Input: part model. Units: mm. Frame: model coordinates. Face numbers are marked on the shaded views. A direction names the side the tool comes from. Round coordinates to 2 decimals unless told otherwise and drop trailing zeros. Loops run counter-clockwise (first coordinate to the right, second up) from the corner with the lowest first, then second, coordinate; pieces in that order, holes last. Notation, with made-up numbers: M -1,46 L 56,46 A24 cw 56,62 Z; hole C 88,22 d4. An arc over 180 degrees is marked long. Put each result on its own line as item: value. Start each with the question number.
1) Pin query (flat end, axial travel): pin 1 (1.9 mm diameter, centred on x = -6, z = -16, fed in from -Y); pin 2 (1.8 mm diameter, centred on y = 2.5, z = -1, fed in from +X); pin 3 (3.5 mm diameter, centred on x = 6, z = -16, fed in from +Y); pin 4 (6 mm diameter, centred on x = -9, z = 7, fed in from +Y). Return the tip coordinate at first contact, or that it passes through.
2) Draft query along Y for the marked faces 4, 5 and 6. Return one class per face: +Y half, -Y half, draft (parallel to the pull), parting line (faces both ways), or undercut.
3) Section B-B on x = 6. Output: boundary loops of the cut face in (y, z).
4) Reachability of the marked faces 1, 2 and 3 from +Z, -Z, +X, -X, +Y, -Y: full face, straight path, thin tool, end or side. Return the list, or none.
5) Section A-A on z = -16. Output: boundary loops of the cut face in (x, y).
6) Line query: probe 1 along X at (y, z) = (-0.55, -16); probe 2 along Z at (x, y) = (6, -0.25); probe 3 along Z at (x, y) = (6.5, 3). Output: solid intervals per line, ascending.
7) Section D-D on y = -0.5. Output: boundary loops of the cut face in (x, z), plus the area to 3 significant figures.
8) Section C-C on x = 3.5. Output: boundary loops of the cut face in (y, z), plus the area to 4 significant figures.
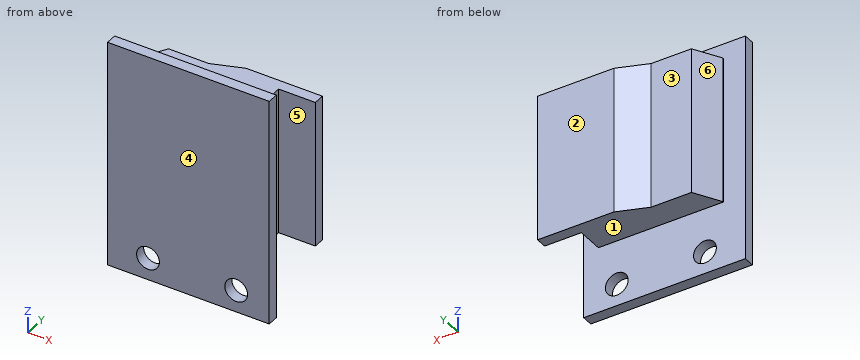
from build123d import *

# Parameters (mm, degrees)
SKIZZE2_W                        = 17
SKIZZE2_H                        = 20
AUFSATZ_LINEAR_AUSTRAGEN1_DEPTH  = 3.6
SKIZZE3_W                        = 22
SKIZZE3_H                        = 31
AUFSATZ_LINEAR_AUSTRAGEN2_DEPTH  = 1.5
F_3_1_3_1_DURCHMESSER_BOHRUNG1_D = 3.1
SKIZZE10_W                       = 10
SKIZZE10_H                       = 20
AUFSATZ_LINEAR_AUSTRAGEN3_DEPTH  = 1.5
FASE4_SIZE                       = 4.5
FASE4_SIZE_2                     = 1.637866054
FASE5_SIZE                       = 3.5
FASE5_SIZE2                      = 2.020725942


with BuildPart() as part:
    # Skizze2 → Aufsatz-Linear austragen1 (new body)
    with BuildSketch(Plane(origin=(0, 0, 0), x_dir=(1, 0, 0), z_dir=(0, 1, 0))):
        Rectangle(SKIZZE2_W, SKIZZE2_H)
    extrude(amount=AUFSATZ_LINEAR_AUSTRAGEN1_DEPTH)

    # Skizze3 → Aufsatz-Linear austragen2 (add)
    with BuildSketch(Plane(origin=(0, 0, 0), x_dir=(-1, 0, 0), z_dir=(0, -1, 0))):
        with Locations((0.5, 3.5)):
            Rectangle(SKIZZE3_W, SKIZZE3_H)
    extrude(amount=AUFSATZ_LINEAR_AUSTRAGEN2_DEPTH)

    # Ø3.1 (3.1) Durchmesser Bohrung1 (through all)
    with Locations(Plane(origin=(0, -1.5, 0), x_dir=(-1, 0, 0), z_dir=(0, -1, 0))):
        with Locations((6, 16), (-6, 16)):
            Hole(F_3_1_3_1_DURCHMESSER_BOHRUNG1_D / 2)

    # Skizze10 → Aufsatz-Linear austragen3 (add)
    with BuildSketch(Plane(origin=(0, 3.6, 0), x_dir=(1, 0, 0), z_dir=(0, 1, 0))):
        with Locations((8.5, 0)):
            Rectangle(SKIZZE10_W, SKIZZE10_H)
    extrude(amount=AUFSATZ_LINEAR_AUSTRAGEN3_DEPTH)

    # Fase4
    # the kernel refuses this chamfer: 4.5, 1.637866054 mm, written as the material it adds along each edge
    with BuildSketch(Plane(origin=(3.5, 3.6, -10), x_dir=(-0.9999130865277315, -0.01318405819864591, 0), z_dir=(0, 0, 1))) as fase4_piece_1_section:
        Polygon((FASE4_SIZE * 0.999913086528, -FASE4_SIZE * 0.0131840581986), (-FASE4_SIZE_2 * 0.0131840582002, -FASE4_SIZE_2 * 0.999913086649), (0, 0), align=None)
    fase4_piece_1 = extrude(amount=20, mode=Mode.PRIVATE)
    fase4_piece_1 = split(fase4_piece_1, bisect_by=Plane(origin=(1.935786974, 5.1, 0), z_dir=(0, -1, 0)), keep=Keep.TOP, mode=Mode.PRIVATE)
    add(fase4_piece_1)

    # Fase5
    fase5_edges = [part.edges().sort_by_distance(p)[0] for p in [
        (-8.5, 3.6, 0),
    ]]
    fase5_side = [part.faces().sort_by_distance(p)[0] for p in [
        (-8.5, 1.8, 0),
    ]]
    chamfer(fase5_edges, length=FASE5_SIZE, length2=FASE5_SIZE2, reference=fase5_side[0])


solid = part.part
Geometry results:
1. pin 1: passes through
1. pin 2: stops at x = 8.5
1. pin 3: stops at y = 0
1. pin 4: stops at y = 3.6
2. face 4: -Y half
2. face 5: undercut
2. face 6: +Y half
3. outline: M -1.5,-19 L 0,-19 L 0,-17.55 L -1.5,-17.55 Z; M -1.5,-14.45 L 0,-14.45 L 0,-10 L 5.1,-10 L 5.1,10 L 0,10 L 0,12 L -1.5,12 Z
4. face 1: -Z, +X, -X, +Y
4. face 2: +Z, -Z, +X, -X, +Y
4. face 3: +Z, -Z, -X, +Y
5. outline: M -11.5,-1.5 L -7.55,-1.5 L -7.55,0 L -11.5,0 Z; M -4.45,-1.5 L 4.45,-1.5 L 4.45,0 L -4.45,0 Z; M 7.55,-1.5 L 10.5,-1.5 L 10.5,0 L 7.55,0 Z
6. probe 1: x = -11.5 to -7.55, -4.45 to 4.45, 7.55 to 10.5
6. probe 2: z = -19 to -17.55, -14.45 to 12
6. probe 3: z = -10 to 10
7. outline: M -11.5,-19 L 10.5,-19 L 10.5,12 L -11.5,12 Z; hole C -6,-16 d3.1; hole C 6,-16 d3.1
7. area: 667 mm²
8. outline: M -1.5,-19 L 0,-19 L 0,-10 L 5.1,-10 L 5.1,10 L 0,10 L 0,12 L -1.5,12 Z
8. area: 148.5 mm²
